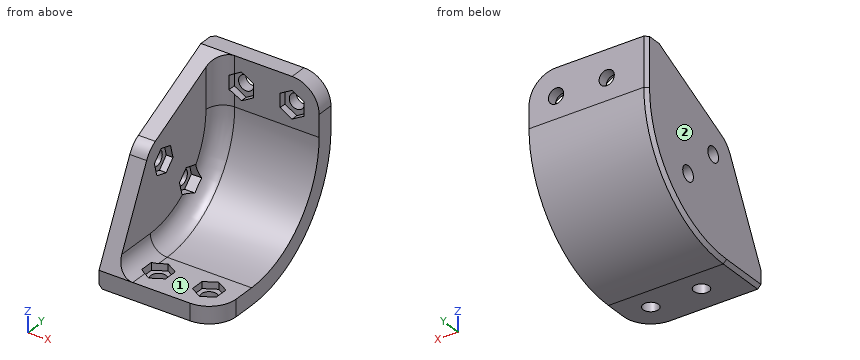
```python
from build123d import *

# Parameters (mm, degrees)
PAD_DEPTH       = 5
PAD001_DEPTH    = 5
PAD002_DEPTH    = 5
FILLET003_R     = 28.5
POCKET003_DEPTH = 35.001
FILLET_R        = 5
SKETCH003_R     = 2.25
HOLE_DEPTH      = 48.001
SKETCH004_R     = 2.25
HOLE001_DEPTH   = 35.001
SKETCH005_R     = 2.25
HOLE002_DEPTH   = 48.001
POCKET_DEPTH    = 2
POCKET001_DEPTH = 2
POCKET002_DEPTH = 2
CHAMFER_SIZE    = 1


with BuildPart() as part:
    # Sketch → Pad (new body)
    with BuildSketch(Plane.YZ):
        with BuildLine():
            Line((0, 48), (-5, 48))
            Line((-31.37532, 35.02115), (-5, 48))
            ThreePointArc((-31.37532, 35.02115), (-33.5, 33.5), (-35.02115, 31.37532))
            Line((-48, 5), (-35.02115, 31.37532))
            Line((-48, 5), (-48, 0))
            Line((-48, 0), (0, 0))
            Line((0, 0), (0, 48))
        make_face()
    extrude(amount=PAD_DEPTH)

    # Sketch001 → Pad001 (join)
    with BuildSketch(Plane.XY):
        with BuildLine():
            Line((0, 0), (0, -48))
            Line((0, -48), (27, -48))
            ThreePointArc((27, -48), (32.656854, -45.656854), (35, -40))
            Line((35, -40), (35, 0))
            Line((35, 0), (0, 0))
        make_face()
    extrude(amount=PAD001_DEPTH)

    # Sketch002 (on DatumPlane) → Pad002 (join)
    with BuildSketch(Plane.XZ):
        with BuildLine():
            Line((0, 0), (0, 48))
            Line((0, 48), (27, 48))
            ThreePointArc((35, 40), (32.656854, 45.656854), (27, 48))
            Line((35, 40), (35, 0))
            Line((35, 0), (0, 0))
        make_face()
    extrude(amount=PAD002_DEPTH)

    # Fillet003
    fillet003_edges = [part.edges().sort_by_distance(p)[0] for p in [
        (20, -5, 5),
    ]]
    fillet(fillet003_edges, radius=FILLET003_R)

    # Sketch009 → Pocket003 (cut, through all)
    with BuildSketch(Plane.YZ):
        with BuildLine():
            ThreePointArc((-33.5, 0), (-9.811923, 9.811923), (0, 33.5))
            Line((0, 33.5), (0, 0))
            Line((-33.5, 0), (0, 0))
        make_face()
    extrude(amount=POCKET003_DEPTH, mode=Mode.SUBTRACT)

    # Fillet
    fillet_edges = [part.edges().sort_by_distance(p)[0] for p in [
        (5, -13.347457, 13.347457),
    ]]
    fillet(fillet_edges, radius=FILLET_R)

    # Sketch003 → Hole (cut, through all)
    with BuildSketch(Plane.XY):
        with Locations((12, -40)):
            Circle(SKETCH003_R)
        with Locations((27, -40)):
            Circle(SKETCH003_R)
    extrude(amount=HOLE_DEPTH, mode=Mode.SUBTRACT)

    # Sketch004 → Hole001 (cut, through all)
    with BuildSketch(Plane.YZ):
        with Locations((-17.236544, 17.236544)):
            Circle(SKETCH004_R)
        with Locations((-27.843146, 27.843146)):
            Circle(SKETCH004_R)
    extrude(amount=HOLE001_DEPTH, mode=Mode.SUBTRACT)

    # Sketch005 (on DatumPlane) → Hole002 (cut, through all)
    with BuildSketch(Plane.XZ):
        with Locations((12, 40)):
            Circle(SKETCH005_R)
        with Locations((27, 40)):
            Circle(SKETCH005_R)
    extrude(amount=HOLE002_DEPTH, mode=Mode.SUBTRACT)

    # Sketch006 (on DatumPlane) → Pocket (cut, symmetric)
    with BuildSketch(Plane.XY.offset(5)):
        Polygon((12, -44.070319), (15.525, -42.03516), (15.525, -37.96484), (12, -35.929681), (8.475, -37.96484), (8.475, -42.03516), align=None)
        Polygon((30.525, -42.03516), (30.525, -37.96484), (27, -35.929681), (23.475, -37.96484), (23.475, -42.03516), (27, -44.070319), align=None)
    extrude(amount=POCKET_DEPTH, both=True, mode=Mode.SUBTRACT)

    # Sketch007 (on DatumPlane) → Pocket001 (cut, symmetric)
    with BuildSketch(Plane.YZ.offset(5)):
        Polygon((-31.774772, 28.896622), (-30.721296, 24.964995), (-26.78967, 23.911519), (-23.911519, 26.78967), (-24.964995, 30.721296), (-28.896622, 31.774772), align=None)
        Polygon((-21.168171, 18.29002), (-20.114694, 14.358394), (-16.183068, 13.304917), (-13.304917, 16.183068), (-14.358394, 20.114694), (-18.29002, 21.168171), align=None)
    extrude(amount=POCKET001_DEPTH, both=True, mode=Mode.SUBTRACT)

    # Sketch008 (on DatumPlane) → Pocket002 (cut, symmetric)
    with BuildSketch(Plane.XZ.offset(5)):
        Polygon((12, 35.929681), (15.525, 37.96484), (15.525, 42.03516), (12, 44.070319), (8.475, 42.03516), (8.475, 37.96484), align=None)
        Polygon((27, 35.929681), (30.525, 37.96484), (30.525, 42.03516), (27, 44.070319), (23.475, 42.03516), (23.475, 37.96484), align=None)
    extrude(amount=POCKET002_DEPTH, both=True, mode=Mode.SUBTRACT)

    # Chamfer
    chamfer_edges = [part.edges().sort_by_distance(p)[0] for p in [
        (0, -9.811923, 9.811923),
    ]]
    chamfer(chamfer_edges, length=CHAMFER_SIZE)


solid = part.part
```
For this review, take the finished solid that the model builds, in its own axes (mm). Face numbers are marked on the shaded views. A direction names the side the tool comes from. Coordinates: 2 decimals unless noted, no trailing zeros. Loops run counter-clockwise (first coordinate to the right, second up) from the corner with the lowest first, then second, coordinate; pieces in that order, holes last. Notation, with made-up numbers: (-21.5, 16.5) - (6.5, 16.5) arc R27 cw to (6.5, 50.5) - close; hole circle Ø11 at (5.5, -4.5). An arc over 180 degrees is marked (long way). Use one line per item in the form item = value. Start each with the question number.
1) To check wall thickness, follow probe 1 along X at (y, z) = (-1.4, 40); probe 2 along X at (y, z) = (-40, 0.8); probe 3 along X at (y, z) = (-18, 19.5). State the ranges of each line that lie inside material, in increasing order. Write a range as from..to.
2) For pin 1 (5.5 mm diameter, centred on x = 12, z = 39.5, fed in from -Y); pin 2 (3.5 mm diameter, centred on x = 28.5, y = -40.5, fed in from +Z); pin 3 (6.5 mm diameter, centred on y = -30, z = 27.5, fed in from +X); pin 4 (2.5 mm diameter, centred on x = 27, z = 40, fed in from +Y), all flat-tipped, find the tip position at first contact; note any pin that passes through.
3) Take a section at B-B (x = 13.5). State the section outline as (y, z) points, plus the area to 3 significant figures.
4) Take a section at C-C (x = 31.5). State the section outline as (y, z) points.
5) For the marked faces 1 and 2, list the 3-axis set-ups (+Z, -Z, +X, -X, +Y, -Y) from which the entire face can be reached by the end or side of a thin tool; tool diameter is ignored.
6) Take a section at A-A (x = 17). State the section outline as (y, z) points, plus the area to 3 significant figures.
From the geometry:
q1.probe_1 = 0..9.75, 14.25..24.75, 29.25..35
q1.probe_2 = 0.2..9.75, 14.25..24.75, 29.25..35
q1.probe_3 = 0..3
q2.pin_1 = -3
q2.pin_2 = 3
q2.pin_3 = 5
q2.pin_4 = through
q3.outline = (-48, 0) - (-41.68, 0) - (-41.68, 3) - (-43.2, 3) - (-43.2, 5) - (-48, 5) - close; (-38.32, 0) - (-33.5, 0) arc R33.5 ccw to (0, 33.5) - (0, 38.32) - (-3, 38.32) - (-3, 36.8) - (-5, 36.8) - (-5, 33.5) arc R28.5 cw to (-33.5, 5) - (-36.8, 5) - (-36.8, 3) - (-38.32, 3) - close; (-5, 43.2) - (-3, 43.2) - (-3, 41.68) - (0, 41.68) - (0, 48) - (-5, 48) - close
q3.area = 343 mm2
q4.outline = (-46.61, 0) - (-33.5, 0) arc R33.5 ccw to (0, 33.5) - (0, 46.61) - (-5, 46.61) - (-5, 33.5) arc R28.5 cw to (-33.5, 5) - (-46.61, 5) - close
q5.face_1 = +Z, +X, -Y
q5.face_2 = +Z, -Z, -X, +Y, -Y
q6.outline = (-48, 0) - (-33.5, 0) arc R33.5 ccw to (0, 33.5) - (0, 48) - (-5, 48) - (-5, 33.5) arc R28.5 cw to (-33.5, 5) - (-48, 5) - close
q6.area = 388 mm2
